Input: part model. Units: mm. Frame: model coordinates. Face numbers are marked on the shaded views. A direction names the side the tool comes from. Give positions to 0.01 mm unless a question says otherwise; leave off trailing zeros. Loops run counter-clockwise (first coordinate to the right, second up) from the corner with the lowest first, then second, coordinate; pieces in that order, holes last. Notation, with made-up numbers: (78, 71.5) - (110, 71.5) arc R21 ccw to (110, 92.5) - close; hole circle Ø9 at (-25.5, -34). An arc over 180 degrees is marked (long way). Answer as a JSON object with one key per item and string values.
from build123d import *


with BuildPart() as part:
    # Esquisse1 → Révolution1 (revolve)
    with BuildSketch(Plane.XY, mode=Mode.PRIVATE) as r_volution1_sk:
        with BuildLine():
            Line((-12, -2), (-15.5, -2))
            Line((-15.5, -2), (-15.5, 0.8))
            Line((-15.5, 0.8), (-11, 0.8))
            Line((-11, 0.8), (-7.5, 4.3))
            Line((-7.5, 4.3), (-6.144916598, 4.3))
            ThreePointArc((-6.144916598, 4.3), (-3.464101615, 6.652067348), (0, 7.5))
            Line((0, 7.5), (0, -14))
            ThreePointArc((0, -14), (-3.070175628, -13.659210139), (-5.990882009, -12.653431659))
            ThreePointArc((-5.990882009, -12.653431659), (-7.30840287, -12.515081442), (-8.423361148, -13.230532377))
            ThreePointArc((-8.423361148, -13.230532377), (-10.650662084, -13.891200373), (-12, -12))
            Line((-12, -12), (-12, -2))
        make_face()
    revolve(r_volution1_sk.sketch.rotate(Axis((0, 7.5, 0), (0, -1, 0)), 270), axis=Axis((0, 7.5, 0), (0, -1, 0)))


solid = part.part
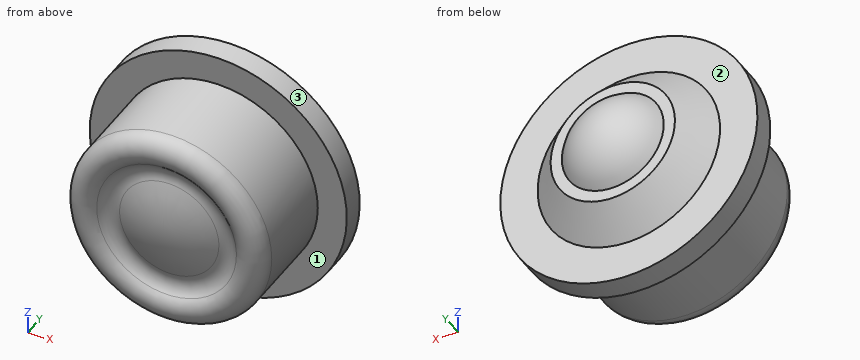
Item 1: Material intervals for line 1 (Z direction, x = -3, y = -5); line 2 (Y direction, x = 6, z = -13); line 3 (Z direction, x = -6, y = -1.75), sorted ascending. Write a range as [from, to].
Geometry check:
{"line 1": "z = [-11.62, 11.62]", "line 2": "y = [-2, 0.8]", "line 3": "z = [-14.29, 14.29]"}
Item 2: Cut plane B-B (x = 0). Return loops of the section in (y, z), then the cut area to 3 significant figures.
Geometry check:
{"outline": "(-13.23, -8.42) arc R2 ccw to (-12, -12) - (-2, -12) - (-2, -15.5) - (0.8, -15.5) - (0.8, -11) - (4.3, -7.5) - (4.3, -6.14) arc R7.5 ccw to (4.3, 6.14) - (4.3, 7.5) - (0.8, 11) - (0.8, 15.5) - (-2, 15.5) - (-2, 12) - (-12, 12) arc R2 ccw to (-13.23, 8.42) arc R2 cw to (-12.65, 5.99) arc R14 ccw to (-12.65, -5.99) arc R2 cw to start", "area": "453 mm2"}
Item 3: Cut plane A-A (z = 0). Return loops of the section in (x, y).
Geometry check:
{"outline": "(-15.5, -2) - (-12, -2) - (-12, -12) arc R2 ccw to (-8.42, -13.23) arc R2 cw to (-5.99, -12.65) arc R14 ccw to (5.99, -12.65) arc R2 cw to (8.42, -13.23) arc R2 ccw to (12, -12) - (12, -2) - (15.5, -2) - (15.5, 0.8) - (11, 0.8) - (7.5, 4.3) - (6.14, 4.3) arc R7.5 ccw to (-6.14, 4.3) - (-7.5, 4.3) - (-11, 0.8) - (-15.5, 0.8) - close"}
Item 4: Contact query for flat-ended pins moving along their axis: P1, Ø2, axis at y = 4, z = 3.5, coming from the -X side; P2, Ø12, axis at x = -4.5, y = -7, coming from the -Z side; P3, Ø9.5, axis at x = -5, z = -1, coming from the -Y side. Output: stop coordinate, or through.
Geometry check:
{"P1": "stops at x = -8.15", "P2": "stops at z = -15.45", "P3": "stops at y = -14"}
Item 5: Cut plane D-D (y = -3.75). Return loops of the section in (x, z).
Geometry check:
{"outline": "circle Ø24 at (0, 0)"}
Item 6: Access query for the marked faces 1, 2 and 3. Directions: +Z, -Z, +X, -X, +Y, -Y. A direction counts if a zero-diameter tool reaches every point of the face in a straight line with its end or side. Return the directions, or none.
Geometry check:
{"face 1": "-Y", "face 2": "+Y", "face 3": "+Y, -Y"}
Item 7: Cut plane C-C (y = 5.5). Return loops of the section in (x, z), then the cut area to 3 significant figures.
Geometry check:
{"outline": "circle Ø10.2 at (0, 0)", "area": "81.7 mm2"}
